```python
from build123d import *

# Parameters (mm, degrees)
SKETCH1_W                 = 48
SKETCH1_H                 = 41
BASE_EXTRUSION_DEPTH      = 15
SKETCH1_14_W              = 6.375
SKETCH1_14_H              = 36
CLEARANCE_EXTENSION_DEPTH = 6.35
F_8_32_TAPPED_HOLE6_D     = 3.4544
F_8_32_TAPPED_HOLE6_DEPTH = 13.96
F_8_32_TAPPED_HOLE6_TIP   = 1.037806461
F_6_32_TAPPED_HOLE1_D     = 2.7051


with BuildPart() as part:
    # Sketch1 → Base Extrusion (new body)
    with BuildSketch(Plane.XY):
        with Locations((1.5, 0)):
            Rectangle(SKETCH1_W, SKETCH1_H)
    extrude(amount=BASE_EXTRUSION_DEPTH)

    # Sketch1<14> → Clearance Extension (add)
    with BuildSketch(Plane.XY):
        with Locations((22.3125, 0)):
            Rectangle(SKETCH1_14_W, SKETCH1_14_H)
    extrude(amount=-CLEARANCE_EXTENSION_DEPTH)

    # #8-32 Tapped Hole6
    with Locations(Plane(origin=(15, 0, 15), x_dir=(1, 0, 0), z_dir=(0, 0, 1))):
        with Locations((0, 0), (-30, 0)):
            Hole(F_8_32_TAPPED_HOLE6_D / 2, depth=F_8_32_TAPPED_HOLE6_DEPTH)
            with Locations((0, 0, -(F_8_32_TAPPED_HOLE6_DEPTH + F_8_32_TAPPED_HOLE6_TIP / 2))):  # 118° drill point
                Cone(0, F_8_32_TAPPED_HOLE6_D / 2, F_8_32_TAPPED_HOLE6_TIP, mode=Mode.SUBTRACT)

    # #6-32 Tapped Hole1 (through all)
    with Locations(Plane(origin=(25.5, 0, 0), x_dir=(0, 0, -1), z_dir=(1, 0, 0))):
        with Locations((3.175, 9.25), (3.175, -9.25)):
            Hole(F_6_32_TAPPED_HOLE1_D / 2)


solid = part.part
```
Check sheet for the modelled part. Datum: model origin and axes. Units: mm. A direction names the side the tool comes from. Round coordinates to 2 decimals unless told otherwise and drop trailing zeros. Order: outer loops, then holes, each group sorted by start corner. A loop starts at its lowest first (then second) coordinate and runs counter-clockwise, first axis right, second up. Notation, with made-up numbers: (52.5, -36) -> (78.5, -36) arc R23 cw to (78.5, -20) -> close; hole circle Ø7 at (14, 12.25). An arc over 180 degrees is marked (long way). One line per item, written item: value. Start each with the question number.
Q1. Cross-section at C-C (y = -16). Record the boundary of the cut face in (x, z) (3 decimals), and give its area (3 significant figures).
Q2. Set-up check for faces 5 (the face through (19.125, 0, -3)), 6 (the face through (22, 18, -3)), 7 (the face through (22, -18, -3)), 8 (the face through (-13.274, 0.076, 7.922)): record each of +Z, -Z, +X, -X, +Y, -Y from which the full face is reachable in a straight line by a thin tool's end or side.
Q3. Cross-section at D-D (x = 9.5). Record the boundary of the cut face in (y, z).
Q4. Gauge pin test, flat ends, axial feed: pin 1 Ø3 at (x, z) = (22, -4.5) entering from +Y; pin 2 Ø7 at (x, z) = (22.5, -4) entering from -Y; pin 3 Ø5.5 at (x, y) = (15, 0) entering from -Z. Record the tip position at first contact, or that the pin passes through.
Q5. Cross-section at B-B (x = 21.5). Record the boundary of the cut face in (y, z) (3 decimals), and give its area (3 significant figures).
Q6. Mould release check, pull along Y, two halves, no side actions. Record for faces 1 (the face through (1, 20.5, 7)), 2 (the face through (16.726, 0.076, 7.922)), 3 (the face through (-22.5, 0, 7)), 4 (the face through (1, -20.5, 7)): pulls with the +Y half, pulls with the -Y half, needs draft (parallel to the pull), parting line crosses it, or undercut.
Q7. Cross-section at A-A (y = -9.25). Record the boundary of the cut face in (x, z) (3 decimals), and give its area (3 significant figures).
Q8. Thickness scan on line 1 (X direction, y = 0, z = 10.25); line 2 (Y direction, x = 15, z = 9.25); line 3 (Z direction, x = -2.5, y = 1.5). Record the ranges inside material, lowest first.
Completed:
1. outline: (-22.5, 0) -> (19.125, 0) -> (19.125, -6.35) -> (25.5, -6.35) -> (25.5, 15) -> (-22.5, 15) -> close
1. area: 760 mm²
2. face 5: -Z, -X, +Y, -Y
2. face 6: -Z, +X, -X, +Y
2. face 7: -Z, +X, -X, -Y
2. face 8: +Z
3. outline: (-20.5, 0) -> (20.5, 0) -> (20.5, 15) -> (-20.5, 15) -> close
4. pin 1: stops at y = 18
4. pin 2: stops at y = -18
4. pin 3: stops at z = 0
5. outline: (-20.5, 0) -> (-18, 0) -> (-18, -6.35) -> (18, -6.35) -> (18, 0) -> (20.5, 0) -> (20.5, 15) -> (-20.5, 15) -> close; hole circle Ø2.705 at (-9.25, -3.175); hole circle Ø2.705 at (9.25, -3.175)
5. area: 832 mm²
6. face 1: pulls with the +Y half
6. face 2: undercut
6. face 3: needs draft
6. face 4: pulls with the -Y half
7. outline: (-22.5, 0) -> (19.125, 0) -> (19.125, -1.822) -> (25.5, -1.822) -> (25.5, 15) -> (-22.5, 15) -> close; (19.125, -6.35) -> (25.5, -6.35) -> (25.5, -4.528) -> (19.125, -4.528) -> close
7. area: 743 mm²
8. line 1: x = -22.5 to -16.73, -13.27 to 13.27, 16.73 to 25.5
8. line 2: y = -20.5 to -1.73, 1.73 to 20.5
8. line 3: z = 0 to 15
